from build123d import *

# Parameters (mm, degrees)
SKETCH1_W           = 18.7
SKETCH1_H           = 64.5
BOSS_EXTRUDE1_DEPTH = 22.5
SKETCH2_R           = 2.7
BOSS_EXTRUDE2_DEPTH = 9


with BuildPart() as part:
    # Sketch1 → Boss-Extrude1 (new body)
    with BuildSketch(Plane(origin=(0, 0, 0), x_dir=(1, 0, 0), z_dir=(0, 1, 0))):
        Rectangle(SKETCH1_W, SKETCH1_H)
    extrude(amount=BOSS_EXTRUDE1_DEPTH)

    # Sketch2 → Boss-Extrude2 (add)
    with BuildSketch(Plane(origin=(9.35, 0, 0), x_dir=(0, 0, -1), z_dir=(1, 0, 0))):
        with Locations((21.05, 11.25)):
            Circle(SKETCH2_R)
    boss_extrude2 = extrude(amount=BOSS_EXTRUDE2_DEPTH)

    # Mirror1: Boss-Extrude2 across plane
    add(boss_extrude2.mirror(Plane(origin=(0, 0, 0), x_dir=(0, 0, 1), z_dir=(1, 0, 0))))


solid = part.part
Model file for the job. Use its own axes, mm. A direction names the side the tool comes from. Coordinates: 2 decimals unless noted, no trailing zeros. Write each loop counter-clockwise with the first axis right and the second up, starting at its lowest first coordinate (ties: lowest second). Pieces come first, ordered by that corner, then holes. Notation, with made-up numbers: (69.25, 12) -> (93.25, 12) arc R23 ccw to (93.25, 41) -> close; hole circle Ø6 at (85, 24.25). An arc over 180 degrees is marked (long way). One line per item, written item: value. Start each with the question number.
1) Slice it at C-C on x = -14. Write the cut outline in (y, z).
2) Slice it at A-A on y = 11.25. Write the cut outline in (x, z), then the cut area to 3 significant figures.
3) Which spindle directions (+Z, -Z, +X, -X, +Y, -Y) get a long thin tool onto all of the face, cutting with end or side? Do faces 1 (the face through (13.787, 13.527, -22.502)), 2 (the face through (-13.787, 13.527, -22.502)), 3 (the face through (0, 11, 32.25)). Say none if no direction does.
4) Slice it at D-D on z = 18. Write the cut outline in (x, y).
5) Probe probe 1 along X at (y, z) = (2.25, -20). List the from-to ranges inside material, lowest first.
6) Flat gauge pins, fed straight in: pin 1 Ø11 at (y, z) = (9, 10) entering from +X; pin 2 Ø8 at (x, z) = (-14, -17.5) entering from +Y; pin 3 Ø6 at (y, z) = (4.5, 17) entering from -X. Where does each tip first touch, or does it go through?
7) Slice it at B-B on z = -21.05. Write the cut outline in (x, y).
Answers follow:
1. outline: circle Ø5.4 at (11.25, -21.05)
2. outline: (-18.35, -23.75) -> (-9.35, -23.75) -> (-9.35, -32.25) -> (9.35, -32.25) -> (9.35, -23.75) -> (18.35, -23.75) -> (18.35, -18.35) -> (9.35, -18.35) -> (9.35, 32.25) -> (-9.35, 32.25) -> (-9.35, -18.35) -> (-18.35, -18.35) -> close
2. area: 1,300 mm2
3. face 1: +X
3. face 2: -X
3. face 3: +Z, +X, -X, +Y, -Y
4. outline: (-9.35, 0) -> (9.35, 0) -> (9.35, 22.5) -> (-9.35, 22.5) -> close
5. probe 1: -9.35 to 9.35
6. pin 1: x = 9.35
6. pin 2: y = 13.95
6. pin 3: x = -9.35
7. outline: (-18.35, 8.55) -> (-9.35, 8.55) -> (-9.35, 0) -> (9.35, 0) -> (9.35, 8.55) -> (18.35, 8.55) -> (18.35, 13.95) -> (9.35, 13.95) -> (9.35, 22.5) -> (-9.35, 22.5) -> (-9.35, 13.95) -> (-18.35, 13.95) -> close
